from build123d import *

# Parameters (mm, degrees)
SKETCH1_W           = 174.625
SKETCH1_H           = 144.4625
SKETCH1_R           = 3.175
BOSS_EXTRUDE1_DEPTH = 6.35
SKETCH2_W           = 23.394418878
SKETCH2_H           = 46.463143603
BOSS_EXTRUDE2_DEPTH = 6.35


with BuildPart() as part:
    # Sketch1 → Boss-Extrude1 (new body)
    with BuildSketch(Plane(origin=(0, 0, 0), x_dir=(0, 0, -1), z_dir=(1, 0, 0))):
        Rectangle(SKETCH1_W, SKETCH1_H)
        with Locations((-55.5625, 55.5625)):
            Circle(SKETCH1_R, mode=Mode.SUBTRACT)
        with Locations((55.5625, 55.5625)):
            Circle(SKETCH1_R, mode=Mode.SUBTRACT)
        with Locations((55.5625, -55.5625)):
            Circle(SKETCH1_R, mode=Mode.SUBTRACT)
        with Locations((-55.5625, -55.5625)):
            Circle(SKETCH1_R, mode=Mode.SUBTRACT)
    extrude(amount=BOSS_EXTRUDE1_DEPTH)

    # Sketch2 → Boss-Extrude2 (add)
    with BuildSketch(Plane.ZY):
        with Locations((73.609709439, 47.837821802)):
            Rectangle(SKETCH2_W, SKETCH2_H)
        with Locations((-73.609709439, 47.837821802)):
            Rectangle(SKETCH2_W, SKETCH2_H)
        with Locations((-73.609709439, -47.837821802)):
            Rectangle(SKETCH2_W, SKETCH2_H)
        with Locations((73.609709439, -47.837821802)):
            Rectangle(SKETCH2_W, SKETCH2_H)
    extrude(amount=BOSS_EXTRUDE2_DEPTH)


solid = part.part
Verification items for the finished model (mm, model axes). A direction names the side the tool comes from. Give positions to 0.01 mm unless a question says otherwise; leave off trailing zeros. Loops run counter-clockwise (first coordinate to the right, second up) from the corner with the lowest first, then second, coordinate; pieces in that order, holes last.
1) Sectioned sample at C-C, the plane y = 50. Enter the section's corners in (x, z), then the cut area to 3 significant figures.
2) Sectioned sample at D-D, the plane y = 0. Enter the section's corners in (x, z).
3) Set-up check for faces 1 (the flat face through (-3, -71.069, 73)), 2 (the flat face through (-3, -24.606, 73)), 3 (the flat face through (-3, 71.069, 73)): record each of +Z, -Z, +X, -X, +Y, -Y from which the full face is reachable in a straight line by a thin tool's end or side.
4) Depth check by flat-ended pin: pin 1 Ø3 at (x, z) = (-3, -68.5) entering from +Y; pin 2 Ø4 at (y, z) = (55.56, 55.56) entering from -X; pin 3 Ø5 at (x, y) = (-3, 48) entering from -Z; pin 4 Ø1.9 at (x, z) = (-3, 74) entering from -Y. Enter the tip coordinate at first touch or a pass-through.
5) Thickness scan on line 1 along Z through (x, y) = (-3, -46); line 2 along Y through (x, z) = (-1.75, 69); line 3 along X through (y, z) = (45, -53). Record the ranges inside material, lowest first.
6) Sectioned sample at A-A, the plane x = -2. Enter the section's corners in (y, z), then the cut area to 3 significant figures.
7) Sectioned sample at B-B, the plane z = -70. Enter the section's corners in (x, y), then the cut area to 3 significant figures.
8) Draft check along Z on faces 4 (the flat face through (-3, -48, -85.307)), 5 (the cylindrical face through (3.131, 52.746, 54.097)), 6 (the flat face through (-3, 24.606, 73)), 7 (the flat face through (-3, 48, 85.307)). Enter one of: pulls with the +Z half, pulls with the -Z half, needs draft (parallel to the pull), parting line crosses it, or undercut.
Answers:
1. outline: (-6.35, -85.31) - (0, -85.31) - (0, -87.31) - (6.35, -87.31) - (6.35, 87.31) - (0, 87.31) - (0, 85.31) - (-6.35, 85.31) - (-6.35, 61.91) - (0, 61.91) - (0, -61.91) - (-6.35, -61.91) - close
1. area: 1,410 mm2
2. outline: (0, -87.31) - (6.35, -87.31) - (6.35, 87.31) - (0, 87.31) - close
3. face 1: +Z, -Z, -X, -Y
3. face 2: +Z, -Z, -X
3. face 3: +Z, -Z, -X, +Y
4. pin 1: stops at y = 71.07
4. pin 2: passes through
4. pin 3: stops at z = -85.31
4. pin 4: stops at y = -71.07
5. line 1: z = -85.31 to -61.91, 61.91 to 85.31
5. line 2: y = -71.07 to -24.61, 24.61 to 71.07
5. line 3: x = 0 to 6.35
6. outline: (-71.07, -85.31) - (-24.61, -85.31) - (-24.61, -61.91) - (-71.07, -61.91) - close; (-71.07, 61.91) - (-24.61, 61.91) - (-24.61, 85.31) - (-71.07, 85.31) - close; (24.61, -85.31) - (71.07, -85.31) - (71.07, -61.91) - (24.61, -61.91) - close; (24.61, 61.91) - (71.07, 61.91) - (71.07, 85.31) - (24.61, 85.31) - close
6. area: 4,350 mm2
7. outline: (-6.35, -71.07) - (0, -71.07) - (0, -72.23) - (6.35, -72.23) - (6.35, 72.23) - (0, 72.23) - (0, 71.07) - (-6.35, 71.07) - (-6.35, 24.61) - (0, 24.61) - (0, -24.61) - (-6.35, -24.61) - close
7. area: 1,510 mm2
8. face 4: pulls with the -Z half
8. face 5: undercut
8. face 6: needs draft
8. face 7: pulls with the +Z half
